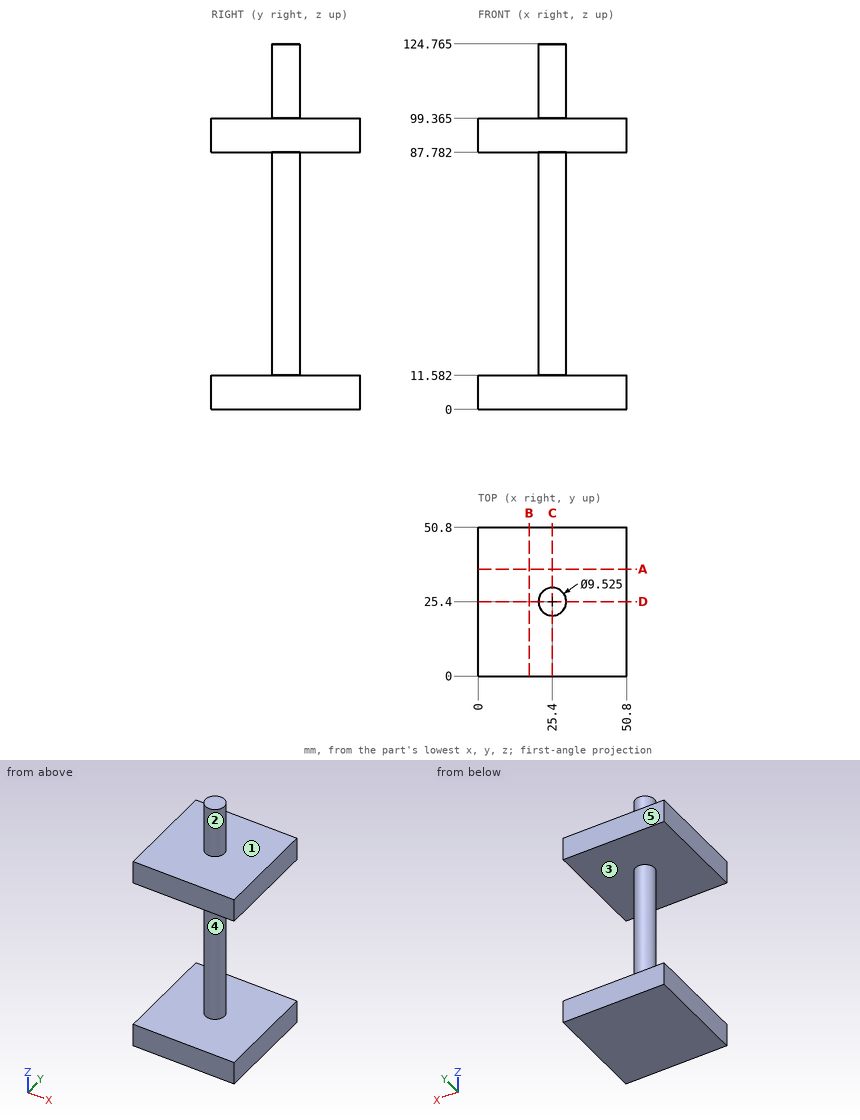
For this review, use the dimensioned drawing (mm, ordinates from the lowest corner) and the shaded views. A direction names the side the tool comes from. Coordinates: 2 decimals unless noted, no trailing zeros. Order: outer loops, then holes, each group sorted by start corner. A loop starts at its lowest first (then second) coordinate and runs counter-clockwise, first axis right, second up. Notation, with made-up numbers: (47.5, 7) - (68.5, 7) arc R10 cw to (68.5, 26) - close; hole circle Ø6 at (23.5, 0.25). An arc over 180 degrees is marked (long way). Answer as a JSON object with one key per item and string values. Group by question number.
1. For probe 1 along Z at (x, y) = (14.5, 37) (1 decimal); probe 2 along X at (y, z) = (24, 12); probe 3 along X at (y, z) = (21, 66) (1 decimal), list the stretches that pass through material, from the lowest coordinate up.
2. We need section C-C on x = 25.4. State the section outline as (y, z) points (1 decimal), then the cut area to 3 significant figures.
3. We need section A-A on y = 36.5. State the section outline as (x, z) points (1 decimal), then the cut area to 3 significant figures.
4. For the marked faces 4 and 5, list the 3-axis set-ups (+Z, -Z, +X, -X, +Y, -Y) from which the entire face can be reached by the end or side of a thin tool; tool diameter is ignored.
5. Clearance check with flat-ended pins moving along their axes: P1, Ø8, axis at x = 27, z = 58, coming from the +Y side; P2, Ø1.5, axis at x = 25.5, z = 32.5, coming from the -Y side. State where each tip first meets the part, or that it passes through.
6. The part is to be moulded in two halves that separate along Z. For the marked faces 1, 2 and 3, say which applies: pulls with the +Z half, pulls with the -Z half, needs draft (parallel to the pull), parting line crosses it, or undercut.
Final values:
{
 "1": {"probe 1": "0 to 11.6, 87.8 to 99.4", "probe 2": "20.85 to 29.95", "probe 3": "23.6 to 27.2"},
 "2": {"outline": "(0, 0) - (50.8, 0) - (50.8, 11.6) - (30.2, 11.6) - (30.2, 87.8) - (50.8, 87.8) - (50.8, 99.4) - (30.2, 99.4) - (30.2, 124.8) - (20.6, 124.8) - (20.6, 99.4) - (0, 99.4) - (0, 87.8) - (20.6, 87.8) - (20.6, 11.6) - (0, 11.6) - close", "area": "2,140 mm²"},
 "3": {"outline": "(0, 0) - (50.8, 0) - (50.8, 11.6) - (0, 11.6) - close; (0, 87.8) - (50.8, 87.8) - (50.8, 99.4) - (0, 99.4) - close", "area": "1,180 mm²"},
 "4": {"face 4": "none", "face 5": "+Z, -Z, +X, -X, +Y"},
 "5": {"P1": "y = 30.16", "P2": "y = 20.64"},
 "6": {"face 1": "pulls with the +Z half", "face 2": "needs draft", "face 3": "undercut"}
}
